For this review, take the finished solid that the model builds, in its own axes (mm). Round coordinates to 2 decimals unless told otherwise and drop trailing zeros. Write each loop counter-clockwise with the first axis right and the second up, starting at its lowest first coordinate (ties: lowest second). Pieces come first, ordered by that corner, then holes.
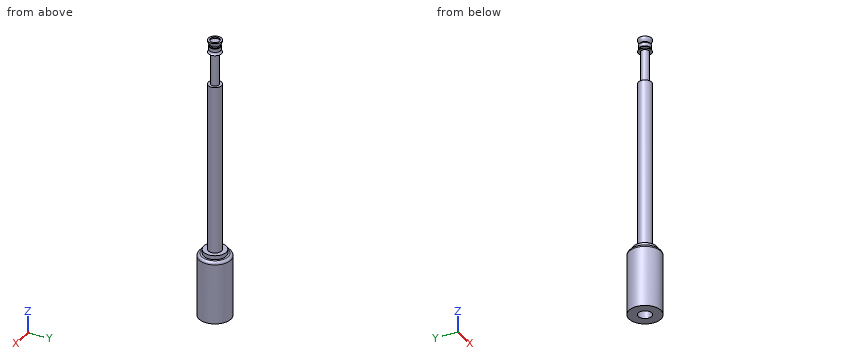
from build123d import *

# Parameters (mm, degrees)
SKETCH1_R           = 12.7
BOSS_EXTRUDE1_DEPTH = 393.7
SKETCH1_3_R         = 30.48
SKETCH1_3_R_2       = 12.7
BOSS_EXTRUDE2_DEPTH = 120.65
FILLET1_R           = 5.08
SKETCH2_R           = 21.59
BOSS_EXTRUDE3_DEPTH = 7.62
SKETCH4_W           = 11.455449348
SKETCH4_H           = 1.487714446
SKETCH5_W           = 19.408085654
SKETCH5_H           = 62.484


with BuildPart() as part:
    # Sketch1 → Boss-Extrude1 (new body)
    with BuildSketch(Plane.XY):
        Circle(SKETCH1_R)
    extrude(amount=BOSS_EXTRUDE1_DEPTH)



with BuildPart() as body_2:
    # Sketch1_3 → Boss-Extrude2 (new body)
    with BuildSketch(Plane.XY):
        Circle(SKETCH1_3_R)
        Circle(SKETCH1_3_R_2, mode=Mode.SUBTRACT)
    extrude(amount=-BOSS_EXTRUDE2_DEPTH)

    # Fillet1
    fillet1_edges = [body_2.edges().sort_by_distance(p)[0] for p in [
        (-30.48, 0, 0),
    ]]
    fillet(fillet1_edges, radius=FILLET1_R)


with BuildPart() as part_1:
    add(part.part)

    add(body_2.part)  # Boss-Extrude3 merges body 2
    # Sketch2 → Boss-Extrude3 (add)
    with BuildSketch(Plane.XY):
        with Locations(Location((0, 0, 0), (0, 0, 180))):
            Circle(SKETCH2_R)
    extrude(amount=BOSS_EXTRUDE3_DEPTH)

    # Sketch3 → Revolve2 (revolve)
    with BuildSketch(Plane(origin=(0, 0, 0), x_dir=(1, 0, 0), z_dir=(0, 1, 0)), mode=Mode.PRIVATE) as revolve2_sk:
        with BuildLine():
            Line((12.7, -393.7), (0, -393.7))
            Line((0, -393.7), (0, -408.3685))
            ThreePointArc((0, -408.3685), (6.286179285, -410.972320715), (8.89, -417.2585))
            Line((8.89, -417.2585), (12.7, -417.2585))
            ThreePointArc((12.7, -417.2585), (11.805440428, -412.576451698), (9.247783259, -408.5539894))
            Line((9.247783259, -408.5539894), (9.247783259, -405.935541368))
            Line((9.247783259, -405.935541368), (10.947551139, -405.935541368))
            Line((10.947551139, -405.935541368), (10.947551139, -399.059207672))
            Line((10.947551139, -399.059207672), (9.170521083, -399.059207672))
            ThreePointArc((9.170521083, -399.059207672), (10.132151594, -395.850690557), (12.7, -393.7))
        make_face()
    revolve(revolve2_sk.sketch.rotate(Axis((0, 0, 393.7), (0, 0, 1)), 180), axis=Axis((0, 0, 393.7), (0, 0, 1)))

    # Sketch4 → Revolve3 (revolve)
    with BuildSketch(Plane(origin=(0, 0, 0), x_dir=(1, 0, 0), z_dir=(0, 1, 0))):
        with Locations((-5.727724674, -414.292142777)):
            Rectangle(SKETCH4_W, SKETCH4_H)
    revolve(axis=Axis((0, 0, 393.7), (0, 0, 1)))

    # Sketch5 → Cut-Revolve1 (revolve, cut)
    with BuildSketch(Plane(origin=(0, 0, 0), x_dir=(1, 0, 0), z_dir=(0, 1, 0)), mode=Mode.PRIVATE) as cut_revolve1_sk:
        with Locations((-17.227522827, -362.458)):
            Rectangle(SKETCH5_W, SKETCH5_H)
    revolve(cut_revolve1_sk.sketch.rotate(Axis((0, 0, 417.2585), (0, 0, -1)), 180), axis=Axis((0, 0, 417.2585), (0, 0, -1)), mode=Mode.SUBTRACT)


solid = part_1.part
(1) We need section A-A, the plane z = -85.5. Give the boundary of the cut face in (x, y).
Geometry check:
outline: circle Ø60.96 at (0, 0); hole circle Ø25.4 at (0, 0)
(2) For pin 1 Ø8 at (x, y) = (1, 1.5) entering from -Z; pin 2 Ø1 at (x, y) = (0, -22.5) entering from +Z; pin 3 Ø17.5 at (x, y) = (-2.5, -5) entering from -Z; pin 4 Ø7.5 at (x, y) = (3, -2) entering from +Z, all flat-tipped, find the tip position at first contact; note any pin that passes through.
Geometry check:
pin 1: stops at z = 0
pin 2: stops at z = 0
pin 3: stops at z = -120.65
pin 4: stops at z = 415.04
(3) For line 1 along Y through (x, z) = (0, -53); line 2 along Z through (x, y) = (-13, 15); line 3 along Z through (x, y) = (24, 2.5), list the stretches that pass through material, from the lowest coordinate up.
Geometry check:
line 1: y = -30.48 to -12.7, 12.7 to 30.48
line 2: z = -120.65 to 7.62
line 3: z = -120.65 to 0
(4) We need section B-B, the plane z = 236. Give the boundary of the cut face in (x, y).
Geometry check:
outline: circle Ø25.4 at (0, 0)
